Can you work these out from the drawing? Everything is in mm from the part's minimum corner. Coordinates: 2 decimals unless noted, no trailing zeros. Order: outer loops, then holes, each group sorted by start corner. A loop starts at its lowest first (then second) coordinate and runs counter-clockwise, first axis right, second up. Notation, with made-up numbers: (44.25, 9) -> (85.25, 9) arc R22 cw to (85.25, 20) -> close; hole circle Ø9 at (16, -18). An arc over 180 degrees is marked (long way). Use a Markdown table: item, result. Add a question column.
1) If we section it at B-B (x = 98.5): Write out the boundary of the cut face in (y, z).
2) If we section it at A-A (z = 1.8): Write out the boundary of the cut face in (x, y), plus the area to 3 significant figures.
3) Will these pins go through, and if not, where does the flat tip stop? pin 1 Ø1.5 at (x, z) = (115, 1) entering from +Y; pin 2 Ø1.2 at (y, z) = (212, 2) entering from +X; pin 3 Ø1.2 at (y, z) = (5, 2.5) entering from +X; pin 4 Ø5 at (x, y) = (260, 205) entering from -Z.
4) If I drill on L1, parallel to Y at x = 10, z = 3.1; L2, parallel to Y at x = 75, z = 0.65, over which ranges is the centre line in solid material (lowest first)? Write a range as [from, to].
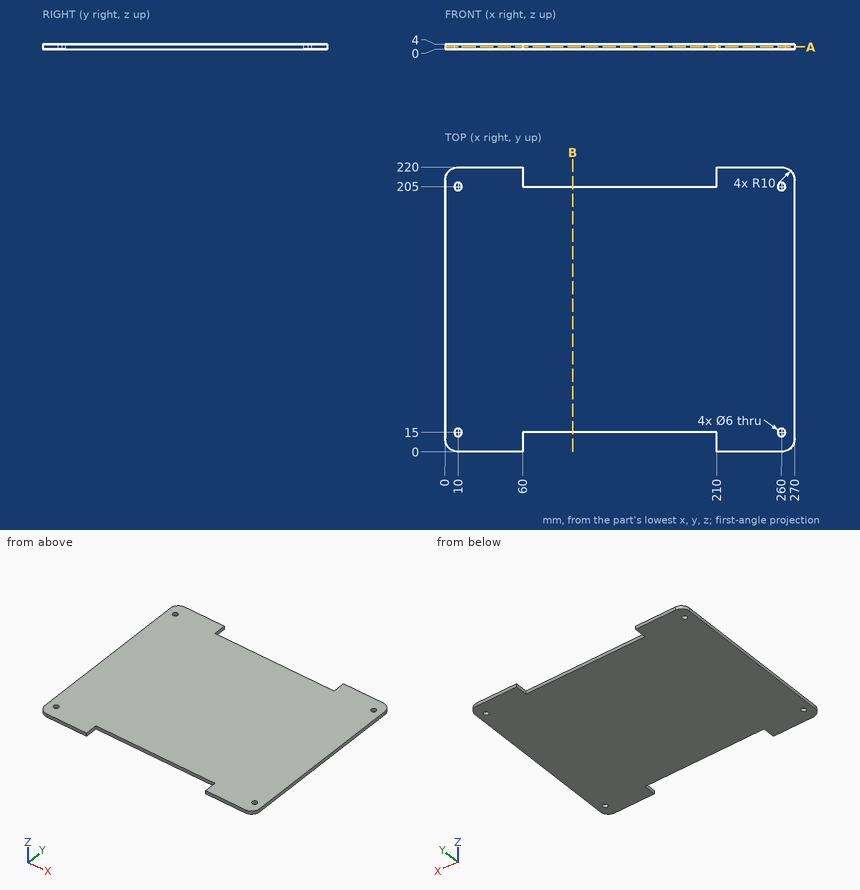
Answer sheet:
| question | item | result |
|---|---|---|
| 1 | outline | (15, 0) -> (205, 0) -> (205, 4) -> (15, 4) -> close |
| 2 | outline | (0, 10) arc R10 ccw to (10, 0) -> (60, 0) -> (60, 15) -> (210, 15) -> (210, 0) -> (260, 0) arc R10 ccw to (270, 10) -> (270, 210) arc R10 ccw to (260, 220) -> (210, 220) -> (210, 205) -> (60, 205) -> (60, 220) -> (10, 220) arc R10 ccw to (0, 210) -> close; hole circle Ø6 at (10, 15); hole circle Ø6 at (10, 205); hole circle Ø6 at (260, 15); hole circle Ø6 at (260, 205) |
| 2 | area | 54,700 mm2 |
| 3 | pin 1 | y = 205 |
| 3 | pin 2 | x = 269.9 |
| 3 | pin 3 | x = 268.98 |
| 3 | pin 4 | through |
| 4 | L1 | [0, 12], [18, 202], [208, 220] |
| 4 | L2 | [15, 205] |
